from build123d import *

# Parameters (mm, degrees)
SKETCH_1_W          = 45
SKETCH_1_H          = 50
EXTRUDE_1_DEPTH     = 3
SKETCH_2_W          = 45
SKETCH_2_H          = 3
EXTRUDE_2_DEPTH     = 41.3
SKETCH_3_R          = 13
SKETCH_3_R_2        = 2.25
CUT_EXTRUDE_1_DEPTH = 78.407299397
SKETCH_4_R          = 3.1
CUT_EXTRUDE_2_DEPTH = 78.069384323


with BuildPart() as part:
    # 草图1 → 凸台-拉伸1 (new body)
    with BuildSketch(Plane.XY):
        with Locations((22.5, 25)):
            Rectangle(SKETCH_1_W, SKETCH_1_H)
    extrude(amount=EXTRUDE_1_DEPTH)

    # 草图2 → 凸台-拉伸2 (add)
    with BuildSketch(Plane(origin=(0, 0, 0), x_dir=(-1, 0, 0), z_dir=(0, 0, -1))):
        with Locations((-22.5, 1.5)):
            Rectangle(SKETCH_2_W, SKETCH_2_H)
    extrude(amount=-EXTRUDE_2_DEPTH)

    # 草图3 → 切除-拉伸1 (cut, through all)
    with BuildSketch(Plane.XY.offset(3)):
        with Locations((22.5, 27.25)):
            Circle(SKETCH_3_R)
        with Locations((22.5, 44.75)):
            Circle(SKETCH_3_R_2)
        with Locations((40, 27.25)):
            Circle(SKETCH_3_R_2)
        with Locations((22.5, 9.75)):
            Circle(SKETCH_3_R_2)
        with Locations((5, 27.25)):
            Circle(SKETCH_3_R_2)
    extrude(amount=-CUT_EXTRUDE_1_DEPTH, mode=Mode.SUBTRACT)

    # 草图4 → 切除-拉伸2 (cut, through all)
    with BuildSketch(Plane(origin=(0, 3, 0), x_dir=(1, 0, 0), z_dir=(0, 1, 0))):
        with Locations(Location((37, -15, 0), (0, 0, 180))):
            Circle(SKETCH_4_R)
        with Locations(Location((37, -33, 0), (0, 0, 180))):
            Circle(SKETCH_4_R)
        with Locations(Location((8, -33, 0), (0, 0, 180))):
            Circle(SKETCH_4_R)
        with Locations(Location((8, -15, 0), (0, 0, 180))):
            Circle(SKETCH_4_R)
    extrude(amount=-CUT_EXTRUDE_2_DEPTH, mode=Mode.SUBTRACT)


solid = part.part
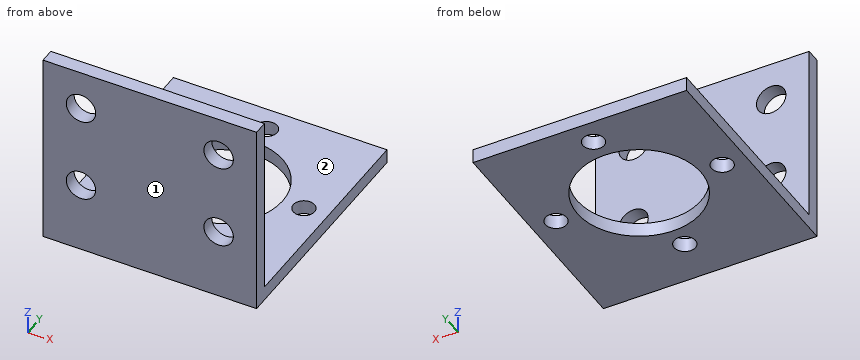
Verification items for the finished model (mm, model axes). Face numbers are marked on the shaded views. A direction names the side the tool comes from. Round coordinates to 2 decimals unless told otherwise and drop trailing zeros. Loops run counter-clockwise (first coordinate to the right, second up) from the corner with the lowest first, then second, coordinate; pieces in that order, holes last. Notation, with made-up numbers: (30, -17.5) - (44, -17.5) arc R13 cw to (44, -6.5) - close; hole circle Ø3 at (5, 66.5). An arc over 180 degrees is marked (long way). Answer in a Markdown table with one row per item. Add a question column.
Q1. Gauge pin test, flat ends, axial feed: pin 1 (7 mm diameter, centred on x = 37, z = 15, fed in from +Y); pin 2 (5 mm diameter, centred on x = 6, z = 26.5, fed in from -Y); pin 3 (22.5 mm diameter, centred on x = 18, y = 19, fed in from +Z). Record the tip position at first contact, or that the pin passes through.
Q2. Material ranges on line 1 (Z direction, x = 37, y = 1.4); line 2 (Z direction, x = 41, y = 8.5), recorded low to high.
Q3. Section check A-A on x = 8. Enter the section's corners in (y, z), plus the area to 3 significant figures.
Q4. Tool access check on the marked faces 1 and 2. Record the directions out of +Z, -Z, +X, -X, +Y, -Y that give a thin tool (end or side, any length) a straight path to the whole face; none if there is none.
Q5. Section check D-D on x = 22.5. Enter the section's corners in (y, z).
Q6. Section check C-C on y = 44.75. Enter the section's corners in (x, z), plus the area to 4 significant figures.
Q7. Section check B-B on z = 33. Enter the section's corners in (x, y).
Found:
| question | item | result |
|---|---|---|
| 1 | pin 1 | stops at y = 3 |
| 1 | pin 2 | stops at y = 0 |
| 1 | pin 3 | stops at z = 3 |
| 2 | line 1 | z = 0 to 11.9, 18.1 to 29.9, 36.1 to 41.3 |
| 2 | line 2 | z = 0 to 3 |
| 3 | outline | (0, 0) - (50, 0) - (50, 3) - (3, 3) - (3, 11.9) - (0, 11.9) - close; (0, 18.1) - (3, 18.1) - (3, 29.9) - (0, 29.9) - close; (0, 36.1) - (3, 36.1) - (3, 41.3) - (0, 41.3) - close |
| 3 | area | 228 mm² |
| 4 | face 1 | +Z, -Z, +X, -X, -Y |
| 4 | face 2 | +Z, +X, -X, +Y |
| 5 | outline | (0, 0) - (7.5, 0) - (7.5, 3) - (3, 3) - (3, 41.3) - (0, 41.3) - close; (12, 0) - (14.25, 0) - (14.25, 3) - (12, 3) - close; (40.25, 0) - (42.5, 0) - (42.5, 3) - (40.25, 3) - close; (47, 0) - (50, 0) - (50, 3) - (47, 3) - close |
| 6 | outline | (0, 0) - (20.25, 0) - (20.25, 3) - (0, 3) - close; (24.75, 0) - (45, 0) - (45, 3) - (24.75, 3) - close |
| 6 | area | 121.5 mm² |
| 7 | outline | (0, 0) - (4.9, 0) - (4.9, 3) - (0, 3) - close; (11.1, 0) - (33.9, 0) - (33.9, 3) - (11.1, 3) - close; (40.1, 0) - (45, 0) - (45, 3) - (40.1, 3) - close |
